Could you check a few things on this model? Use its own coordinates, in mm. A direction names the side the tool comes from. Round coordinates to 2 decimals unless told otherwise and drop trailing zeros. Loops run counter-clockwise (first coordinate to the right, second up) from the corner with the lowest first, then second, coordinate; pieces in that order, holes last. Notation, with made-up numbers: M 76,68.5 L 96,68.5 A18 cw 96,75.5 Z; hole C 61,-16.75 d10. An arc over 180 degrees is marked long. Answer in a Markdown table with one row per item.
```python
from build123d import *

# Parameters (mm, degrees)
BOSS_EXTRUDE1_DEPTH = 0.79375
BOSS_EXTRUDE2_DEPTH = 3.5


with BuildPart() as part:
    # Sketch1 → Boss-Extrude1 (new body)
    with BuildSketch(Plane(origin=(0, 0, 0), x_dir=(1, 0, 0), z_dir=(0, 1, 0))):
        with BuildLine():
            Line((-18.5, 18.5), (18.5, 18.5))
            Line((18.5, 18.5), (18.5, 16.75))
            ThreePointArc((18.5, 16.75), (17.625, 15.875), (18.5, 15))
            Line((18.5, 15), (18.5, -18.5))
            Line((18.5, -18.5), (-18.5, -18.5))
            Line((-18.5, -18.5), (-18.5, 15))
            ThreePointArc((-18.5, 15), (-17.625, 15.875), (-18.5, 16.75))
            Line((-18.5, 16.75), (-18.5, 18.5))
        make_face()
    extrude(amount=BOSS_EXTRUDE1_DEPTH)

    # Sketch2 → Boss-Extrude2 (add)
    with BuildSketch(Plane(origin=(0, 0.79375, 0), x_dir=(1, 0, 0), z_dir=(0, 1, 0))):
        with BuildLine():
            Line((-11.75, 14.5), (11.75, 14.5))
            ThreePointArc((11.75, 14.5), (13.517766953, 13.767766953), (14.25, 12))
            Line((14.25, 12), (14.25, -12))
            ThreePointArc((14.25, -12), (13.517766953, -13.767766953), (11.75, -14.5))
            Line((11.75, -14.5), (-11.75, -14.5))
            ThreePointArc((-11.75, -14.5), (-13.517766953, -13.767766953), (-14.25, -12))
            Line((-14.25, -12), (-14.25, 12))
            ThreePointArc((-14.25, 12), (-13.517766953, 13.767766953), (-11.75, 14.5))
        make_face()
    extrude(amount=BOSS_EXTRUDE2_DEPTH)


solid = part.part
```
1) I need wall thicknesses on line 1 (Z direction, x = 11, y = 3.75); line 2 (Y direction, x = 15, z = 10); line 3 (X direction, y = 3.95, z = 5). Which ranges of each line are inside material? Lowest first, please.
Computed:
| item | result |
|---|---|
| line 1 | z = -14.5 to 14.5 |
| line 2 | y = 0 to 0.79 |
| line 3 | x = -14.25 to 14.25 |
2) I want a section at B-B, the plane z = -11.5. Please give me the cut outline in (x, y), plus the area to 3 significant figures.
Computed:
| item | result |
|---|---|
| outline | M -18.5,0 L 18.5,0 L 18.5,0.79 L 14.25,0.79 L 14.25,4.29 L -14.25,4.29 L -14.25,0.79 L -18.5,0.79 Z |
| area | 129 mm² |
3) I want a section at C-C, the plane x = -15. Please give me the cut outline in (y, z), plus the area to 3 significant figures.
Computed:
| item | result |
|---|---|
| outline | M 0,-18.5 L 0.79,-18.5 L 0.79,18.5 L 0,18.5 Z |
| area | 29.4 mm² |
4) Which directions (+Z, -Z, +X, -X, +Y, -Y) give clear straight access to the entire face, cutting with the end or side of a thin tool? Please do faces 4 (the face through (-14.25, 3, 0)), 5 (the face through (-13.537, 2.519, -13.748)), 6 (the face through (0, 3, -14.5)), 7 (the face through (13.498, 2.519, -13.787)), 8 (the face through (14.25, 3, 0)).
Computed:
| item | result |
|---|---|
| face 4 | +Z, -Z, -X, +Y |
| face 5 | -Z, -X, +Y |
| face 6 | -Z, +X, -X, +Y |
| face 7 | -Z, +X, +Y |
| face 8 | +Z, -Z, +X, +Y |
5) Will these pins go through, and if not, where does the flat tip stop? P1, Ø12, axis at x = 13, z = 9, coming from the -Y side; P2, Ø1, axis at y = 2.5, z = -4.5, coming from the -X side; P3, Ø1.8, axis at y = 3, z = -4, coming from the +X side; P4, Ø2, axis at x = -6.5, y = 2.5, coming from the -Z side.
Computed:
| item | result |
|---|---|
| P1 | stops at y = 0 |
| P2 | stops at x = -14.25 |
| P3 | stops at x = 14.25 |
| P4 | stops at z = -14.5 |
6) If we mould it in two halves opening along Z, with no side actions, what happens to faces 1 (the face through (17.625, 0.391, -15.894)), 2 (the face through (-13.498, 2.519, 13.787)), 3 (the face through (17, 0.794, 0))? For each: released by +Z, released by -Z, zero draft, split by the parting line, or undercut.
Computed:
| item | result |
|---|---|
| face 1 | undercut |
| face 2 | released by +Z |
| face 3 | zero draft |
7) I want a section at A-A, the plane x = -6. Please give me the cut outline in (y, z), plus the area to 3 significant figures.
Computed:
| item | result |
|---|---|
| outline | M 0,-18.5 L 0.79,-18.5 L 0.79,-14.5 L 4.29,-14.5 L 4.29,14.5 L 0.79,14.5 L 0.79,18.5 L 0,18.5 Z |
| area | 131 mm² |
